Verification items for the finished model (mm, model axes). A direction names the side the tool comes from. Give positions to 0.01 mm unless a question says otherwise; leave off trailing zeros. Order: outer loops, then holes, each group sorted by start corner. A loop starts at its lowest first (then second) coordinate and runs counter-clockwise, first axis right, second up. Notation, with made-up numbers: (78, 84) - (122, 84) arc R34 ccw to (122, 114) - close; hole circle Ø4 at (80.25, 6). An arc over 180 degrees is marked (long way). Answer as a JSON object with one key per item and string values. Group by question number.
(1) Mould release check, pull along X, two halves, no side actions. Record for faces 1 (the face through (0, 10, -39)), 2 (the face through (-27.94, 31, 0)), 3 (the face through (25.4, 31, 1)), 4 (the face through (0.32, 64.54, -39.21)): +X half, -X half, draft (parallel to the pull), parting line (faces both ways), or undercut.
(2) Thickness scan on line 1 (Z direction, x = -6.5, y = 50.5); line 2 (X direction, y = 33, z = 28.5); line 3 (Y direction, x = -9.5, z = -32). Record the ranges inside material, lowest first.
(3) Depth check by flat-ended pin: pin 1 Ø15 at (x, z) = (0, 15.24) entering from -Y; pin 2 Ø15 at (x, z) = (-5.5, 13.5) entering from -Y. Enter the tip coordinate at first touch or a pass-through.
(4) Section check A-A (z = 15.24). Record the boundary of the cut face in (x, y), then the cut area to 3 significant figures.
(5) Access from +Z, -Z, +X, -X, +Y, -Y to the whole of each face (thin tool, end or side, straight path). Record for faces 5 (the face through (-26.51, 64.54, -0.5)), 6 (the face through (0, 63.5, 1)).
(6) Section check D-D (y = 6). Record the boundary of the cut face in (x, z), then the cut area to 3 significant figures.
(7) Section check B-B (x = -4). Record the boundary of the cut face in (y, z).
(8) Section check C-C (y = 59). Record the boundary of the cut face in (x, z).
```python
from build123d import *

# Parameters (mm, degrees)
SKETCH2_W                = 55.88
SKETCH2_H                = 81.28
SKETCH2_W_2              = 50.8
SKETCH2_H_2              = 76.2
BOSS_EXTRUDE1_DEPTH      = 63.5
BOSS_EXTRUDE2_DEPTH      = 27.94
BOSS_EXTRUDE2_DEPTH_BACK = 27.94
SKETCH3_W                = 81.28
SKETCH3_H                = 2.54
FILLET1_R                = 5
FILLET4_R                = 5
FILLET5_R                = 5
FILLET6_R                = 5
FILLET7_R                = 5
CUT_EXTRUDE1_REACH       = 84.423
SKETCH4_R                = 5
SKETCH4_R_2              = 9.5
CUT_EXTRUDE2_REACH       = 110.39
SKETCH6_R                = 10


with BuildPart() as part:
    # Sketch2 → Boss-Extrude1 (new body)
    with BuildSketch(Plane(origin=(0, 0, 0), x_dir=(1, 0, 0), z_dir=(0, 1, 0))):
        Rectangle(SKETCH2_W, SKETCH2_H)
        Rectangle(SKETCH2_W_2, SKETCH2_H_2, mode=Mode.SUBTRACT)
    extrude(amount=BOSS_EXTRUDE1_DEPTH)

    # Sketch3 → Boss-Extrude2 (add, two sides: drawn at the far end of the back side and taken through both)
    with BuildSketch(Plane(origin=(0, 0, 0), x_dir=(0, 0, -1), z_dir=(1, 0, 0)).offset(-BOSS_EXTRUDE2_DEPTH_BACK)):
        with Locations((0, 64.77)):
            Rectangle(SKETCH3_W, SKETCH3_H)
    extrude(amount=BOSS_EXTRUDE2_DEPTH + BOSS_EXTRUDE2_DEPTH_BACK)

    # Fillet1
    fillet1_edges = [part.edges().sort_by_distance(p)[0] for p in [
        (0, 66.04, 40.64),
        (0, 66.04, -40.64),
        (-27.94, 66.04, 0),
        (27.94, 66.04, 0),
    ]]
    fillet(fillet1_edges, radius=FILLET1_R)

    # Fillet4
    # the kernel refuses this fillet: 5 mm, written as the material it takes off along each edge
    with BuildSketch(Plane(origin=(-22.94, 61.04, -35.64), x_dir=(-1, 0, 0), z_dir=(0, 0, -1))) as fillet4_piece_1_section:
        Polygon((0, 0), (FILLET4_R, 0), (FILLET4_R, FILLET4_R), (0, FILLET4_R), align=None)
    fillet4_piece_1 = extrude(amount=FILLET4_R, mode=Mode.PRIVATE)
    fillet4_piece_1 = fillet4_piece_1 - Plane(origin=(-22.94, 61.04, -35.64), x_dir=(0.7071067811865475, -0.7071067811865475, 0), z_dir=(0, 0, -1)) * Sphere(FILLET4_R, mode=Mode.PRIVATE)
    add(fillet4_piece_1, mode=Mode.SUBTRACT)
    with BuildSketch(Plane(origin=(-27.94, -12.5, -40.64), x_dir=(1, 0, 0), z_dir=(0, 1, 0))) as fillet4_piece_2:
        with BuildLine():
            CenterArc((FILLET4_R, -FILLET4_R), FILLET4_R, 90, 90)
            Line((0, -FILLET4_R), (0, 0))
            Line((0, 0), (FILLET4_R, 0))
        make_face()
    extrude(amount=73.54, mode=Mode.SUBTRACT)

    # Fillet5
    # the kernel refuses this fillet: 5 mm, written as the material it takes off along each edge
    with BuildSketch(Plane(origin=(22.94, 61.04, -35.64), x_dir=(1, 0, 0), z_dir=(0, 0, -1))) as fillet5_piece_1_section:
        Polygon((0, 0), (FILLET5_R, 0), (FILLET5_R, -FILLET5_R), (0, -FILLET5_R), align=None)
    fillet5_piece_1 = extrude(amount=FILLET5_R, mode=Mode.PRIVATE)
    fillet5_piece_1 = fillet5_piece_1 - Plane(origin=(22.94, 61.04, -35.64), x_dir=(-0.7071067811865475, -0.7071067811865475, 0), z_dir=(0, 0, -1)) * Sphere(FILLET5_R, mode=Mode.PRIVATE)
    add(fillet5_piece_1, mode=Mode.SUBTRACT)
    with BuildSketch(Plane(origin=(27.94, 61.04, -40.64), x_dir=(-1, 0, 0), z_dir=(0, -1, 0))) as fillet5_piece_2:
        with BuildLine():
            CenterArc((FILLET5_R, -FILLET5_R), FILLET5_R, 90, 90)
            Line((0, -FILLET5_R), (0, 0))
            Line((0, 0), (FILLET5_R, 0))
        make_face()
    extrude(amount=73.54, mode=Mode.SUBTRACT)

    # Fillet6
    # the kernel refuses this fillet: 5 mm, written as the material it takes off along each edge
    with BuildSketch(Plane(origin=(22.94, 61.04, 35.64), x_dir=(1, 0, 0), z_dir=(0, 0, 1))) as fillet6_piece_1_section:
        Polygon((0, 0), (FILLET6_R, 0), (FILLET6_R, FILLET6_R), (0, FILLET6_R), align=None)
    fillet6_piece_1 = extrude(amount=FILLET6_R, mode=Mode.PRIVATE)
    fillet6_piece_1 = fillet6_piece_1 - Plane(origin=(22.94, 61.04, 35.64), x_dir=(-0.7071067811865475, -0.7071067811865475, 0), z_dir=(0, 0, 1)) * Sphere(FILLET6_R, mode=Mode.PRIVATE)
    add(fillet6_piece_1, mode=Mode.SUBTRACT)
    with BuildSketch(Plane(origin=(27.94, 61.04, 40.64), x_dir=(-1, 0, 0), z_dir=(0, -1, 0))) as fillet6_piece_2:
        with BuildLine():
            CenterArc((FILLET6_R, FILLET6_R), FILLET6_R, 180, 90)
            Line((0, FILLET6_R), (0, 0))
            Line((0, 0), (FILLET6_R, 0))
        make_face()
    extrude(amount=73.54, mode=Mode.SUBTRACT)

    # Fillet7
    # the kernel refuses this fillet: 5 mm, written as the material it takes off along each edge
    with BuildSketch(Plane(origin=(-22.94, 61.04, 35.64), x_dir=(-1, 0, 0), z_dir=(0, 0, 1))) as fillet7_piece_1_section:
        Polygon((0, 0), (FILLET7_R, 0), (FILLET7_R, -FILLET7_R), (0, -FILLET7_R), align=None)
    fillet7_piece_1 = extrude(amount=FILLET7_R, mode=Mode.PRIVATE)
    fillet7_piece_1 = fillet7_piece_1 - Plane(origin=(-22.94, 61.04, 35.64), x_dir=(0.7071067811865475, -0.7071067811865475, 0), z_dir=(0, 0, 1)) * Sphere(FILLET7_R, mode=Mode.PRIVATE)
    add(fillet7_piece_1, mode=Mode.SUBTRACT)
    with BuildSketch(Plane(origin=(-27.94, -12.5, 40.64), x_dir=(1, 0, 0), z_dir=(0, 1, 0))) as fillet7_piece_2:
        with BuildLine():
            CenterArc((FILLET7_R, FILLET7_R), FILLET7_R, 180, 90)
            Line((0, FILLET7_R), (0, 0))
            Line((0, 0), (FILLET7_R, 0))
        make_face()
    extrude(amount=73.54, mode=Mode.SUBTRACT)

    # Sketch4 → Cut-Extrude1 (cut, up to next)
    with BuildSketch(Plane(origin=(0, 0, 0), x_dir=(1, 0, 0), z_dir=(0, 1, 0)), mode=Mode.PRIVATE) as cut_extrude1_sk1:
        with Locations(Location((0, 15.24, 0), (0, 0, 90))):
            Circle(SKETCH4_R)
    cut_extrude1_tool1 = extrude(cut_extrude1_sk1.sketch, amount=CUT_EXTRUDE1_REACH, mode=Mode.PRIVATE) & part.part
    # Sketch4 → Cut-Extrude1 (cut, up to next)
    with BuildSketch(Plane(origin=(0, 0, 0), x_dir=(1, 0, 0), z_dir=(0, 1, 0)), mode=Mode.PRIVATE) as cut_extrude1_sk2:
        with Locations(Location((0, -15.24, 0), (0, 0, 90))):
            Circle(SKETCH4_R_2)
    cut_extrude1_tool2 = extrude(cut_extrude1_sk2.sketch, amount=CUT_EXTRUDE1_REACH, mode=Mode.PRIVATE) & part.part
    add(cut_extrude1_tool1.solids().sort_by_distance((0, 0, -15.24))[0], mode=Mode.SUBTRACT)
    add(cut_extrude1_tool2.solids().sort_by_distance((0, 0, 15.24))[0], mode=Mode.SUBTRACT)

    # Sketch6 → Cut-Extrude2 (cut, up to next)
    with BuildSketch(Plane(origin=(0, 0, -40.64), x_dir=(-1, 0, 0), z_dir=(0, 0, -1)), mode=Mode.PRIVATE) as cut_extrude2_sk1:
        Circle(SKETCH6_R)
    cut_extrude2_tool1 = extrude(cut_extrude2_sk1.sketch, amount=-CUT_EXTRUDE2_REACH, mode=Mode.PRIVATE) & part.part
    add(cut_extrude2_tool1.solids().sort_by_distance((0, 0, -40.64))[0], mode=Mode.SUBTRACT)


solid = part.part
```
Solutions:
{
 "1": {"face 1": "undercut", "face 2": "-X half", "face 3": "undercut", "face 4": "draft"},
 "2": {"line 1": "z = -40.64 to -38.1, 38.1 to 40.64", "line 2": "x = -27.94 to -25.4, 25.4 to 27.94", "line 3": "y = 63.5 to 66.04"},
 "3": {"pin 1": "passes through", "pin 2": "stops at y = 63.5"},
 "4": {"outline": "(-27.94, 0) - (-25.4, 0) - (-25.4, 63.5) - (-9.5, 63.5) - (-9.5, 66.04) - (-22.94, 66.04) arc R5 ccw to (-27.94, 61.04) - close; (9.5, 63.5) - (25.4, 63.5) - (25.4, 0) - (27.94, 0) - (27.94, 61.04) arc R5 ccw to (22.94, 66.04) - (9.5, 66.04) - close", "area": "406 mm2"},
 "5": {"face 5": "+Z, -Z, -X, +Y", "face 6": "-Y"},
 "6": {"outline": "(-27.94, -35.64) arc R5 ccw to (-22.94, -40.64) - (-8, -40.64) - (-8, -38.1) - (-25.4, -38.1) - (-25.4, 38.1) - (25.4, 38.1) - (25.4, -38.1) - (8, -38.1) - (8, -40.64) - (22.94, -40.64) arc R5 ccw to (27.94, -35.64) - (27.94, 35.64) arc R5 ccw to (22.94, 40.64) - (-22.94, 40.64) arc R5 ccw to (-27.94, 35.64) - close", "area": "609 mm2"},
 "7": {"outline": "(0, 38.1) - (63.5, 38.1) - (63.5, 23.86) - (66.04, 23.86) - (66.04, 35.64) arc R5 ccw to (61.04, 40.64) - (0, 40.64) - close; (9.17, -40.64) - (61.04, -40.64) arc R5 ccw to (66.04, -35.64) - (66.04, -18.24) - (63.5, -18.24) - (63.5, -38.1) - (9.17, -38.1) - close; (63.5, -12.24) - (66.04, -12.24) - (66.04, 6.62) - (63.5, 6.62) - close"},
 "8": {"outline": "(-27.94, -35.64) arc R5 ccw to (-22.94, -40.64) - (22.94, -40.64) arc R5 ccw to (27.94, -35.64) - (27.94, 35.64) arc R5 ccw to (22.94, 40.64) - (-22.94, 40.64) arc R5 ccw to (-27.94, 35.64) - close; hole (-25.4, -38.1) - (25.4, -38.1) - (25.4, 38.1) - (-25.4, 38.1) - close"}
}
